from build123d import *

# Parameters (mm, degrees)
SKETCH2_R               = 10.795
SKETCH2_R_2             = 7.62
BOSS_EXTRUDE1_DEPTH     = 2.2225
SKETCH2_4_R             = 9.652
SKETCH2_4_R_2           = 8.763
BOSS_EXTRUDE2_DEPTH     = 12.7
CUT_EXTRUDE1_DEPTH      = 12.7
CUT_EXTRUDE1_DEPTH_BACK = 12.7
CUT_EXTRUDE2_DEPTH      = 12.7
CUT_EXTRUDE2_DEPTH_BACK = 12.7


with BuildPart() as part:
    # Sketch2 → Boss-Extrude1 (new body)
    with BuildSketch(Plane.XY):
        Circle(SKETCH2_R)
        with Locations((-1.143, 0)):
            Circle(SKETCH2_R_2, mode=Mode.SUBTRACT)
    extrude(amount=BOSS_EXTRUDE1_DEPTH)

    # Sketch2_4 → Boss-Extrude2 (add)
    with BuildSketch(Plane.XY):
        Circle(SKETCH2_4_R)
        Circle(SKETCH2_4_R_2, mode=Mode.SUBTRACT)
    extrude(amount=-BOSS_EXTRUDE2_DEPTH)

    # Sketch3 → Cut-Extrude1 (cut, two sides: drawn at the far end of the back side and taken through both)
    with BuildSketch(Plane(origin=(0, 0, 0), x_dir=(1, 0, 0), z_dir=(0, 1, 0)).offset(-CUT_EXTRUDE1_DEPTH_BACK)):
        Polygon((0, 0), (3.175, 12.7), (-3.175, 12.7), align=None)
    extrude(amount=CUT_EXTRUDE1_DEPTH + CUT_EXTRUDE1_DEPTH_BACK, mode=Mode.SUBTRACT)

    # Sketch5 → Cut-Extrude2 (cut, two sides: drawn at the far end of the back side and taken through both)
    with BuildSketch(Plane(origin=(0, 0, 0), x_dir=(0, 0, -1), z_dir=(1, 0, 0)).offset(-CUT_EXTRUDE2_DEPTH_BACK)):
        Polygon((0, 0), (12.7, 3.175), (12.7, -3.175), align=None)
    extrude(amount=CUT_EXTRUDE2_DEPTH + CUT_EXTRUDE2_DEPTH_BACK, mode=Mode.SUBTRACT)


solid = part.part
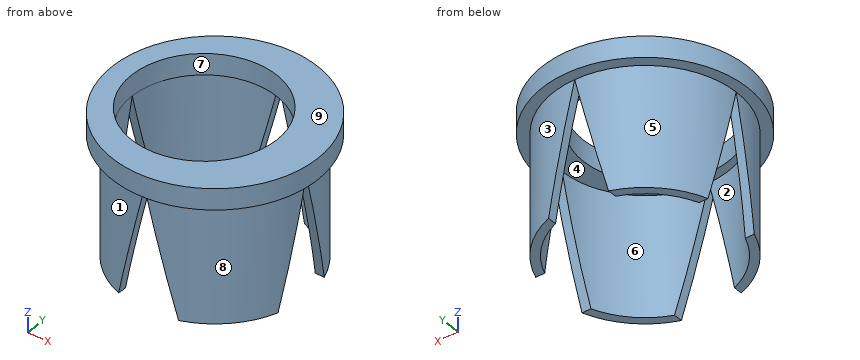
Check sheet for the modelled part. Datum: model origin and axes. Units: mm. Face numbers are marked on the shaded views. A direction names the side the tool comes from. Round coordinates to 2 decimals unless told otherwise and drop trailing zeros. Loops run counter-clockwise (first coordinate to the right, second up) from the corner with the lowest first, then second, coordinate; pieces in that order, holes last. Notation, with made-up numbers: M 6.5,16.25 L 63.5,16.25 A29 ccw 63.5,39.25 Z; hole C -36,2 d9. An arc over 180 degrees is marked long. One line per question, with ' | ' between items. Start each with the question number.
Item 1: Gauge pin test, flat ends, axial feed: pin 1 Ø1 at (x, y) = (6, 4) entering from -Z; pin 2 Ø1.5 at (x, y) = (-3.5, 5.5) entering from -Z; pin 3 Ø5 at (y, z) = (-3.5, -5) entering from -X. Record the tip position at first contact, or that the pin passes through.
Item 2: Set-up check for the marked faces 5, 6, 7, 8 and 9: record each of +Z, -Z, +X, -X, +Y, -Y from which the full face is reachable in a straight line by a thin tool's end or side.
Item 3: Release check for a two-part mould opening along X. For the marked faces 1, 2, 3 and 4 record: released by +X, released by -X, zero draft, split by the parting line, or undercut.
Item 4: Section check D-D (z = 1). Record the boundary of the cut face in (x, y) (3 decimals), and give its area (3 significant figures).
Item 5: Section check B-B (y = -2.5). Record the boundary of the cut face in (x, z), and give its area (3 significant figures).
Item 6: Section check C-C (z = -3.5). Record the boundary of the cut face in (x, y) (3 decimals), and give its area (3 significant figures).
Item 7: Section check A-A (x = -6.5). Record the boundary of the cut face in (y, z), and give its area (3 significant figures).
Item 8: Scan lines: probe 1 along Z at (x, y) = (6.75, -1.5); probe 2 along Y at (x, z) = (3, -2.5); probe 3 along Y at (x, z) = (6.5, -10.25). Record each from-to range of solid material in increasing order.
Worked out:
1) pin 1: z = 0 | pin 2: through | pin 3: x = -9.59
2) face 5: -Z, -X, +Y | face 6: -Z | face 7: +Z, -Z | face 8: -Z, +X, -Y | face 9: +Z, +X, -X, +Y, -Y
3) face 1: released by -X | face 2: undercut | face 3: released by +X | face 4: undercut
4) outline: C 0,0 d21.59; hole C -1.143,0 d15.24 | area: 184 mm^2
5) outline: M -10.5,0 L -9.32,0 L -9.32,-10 L -8.4,-10 L -8.4,0 L -8.34,0 L -8.34,2.22 L -10.5,2.22 Z; M 6.06,0 L 8.4,0 L 8.4,-10 L 9.32,-10 L 9.32,0 L 10.5,0 L 10.5,2.22 L 6.06,2.22 Z | area: 33.2 mm^2
6) outline: M -9.612,-0.875 A9.652 ccw -0.875,-9.612 L -0.875,-8.719 A8.763 cw -8.719,-0.875 Z; M -9.612,0.875 L -8.719,0.875 A8.763 cw -0.875,8.719 L -0.875,9.612 A9.652 ccw Z; M 0.875,-9.612 A9.652 ccw 9.612,-0.875 L 8.719,-0.875 A8.763 cw 0.875,-8.719 Z; M 0.875,8.719 A8.763 cw 8.719,0.875 L 9.612,0.875 A9.652 ccw 0.875,9.612 Z | area: 45.2 mm^2
7) outline: M -8.62,0 L -7.14,0 L -7.14,-12.7 L -5.88,-12.7 L -5.88,0 L -5.42,0 L -5.42,2.22 L -8.62,2.22 Z; M 5.42,0 L 5.88,0 L 5.88,-12.7 L 7.14,-12.7 L 7.14,0 L 8.62,0 L 8.62,2.22 L 5.42,2.22 Z | area: 46.2 mm^2
8) probe 1: 0 to 2.22 | probe 2: -9.17 to -8.23, 8.23 to 9.17 | probe 3: -7.14 to -5.88, 5.88 to 7.14
